from build123d import *

# Parameters (mm, degrees)
F2_DEPTH = 19.05
F3_W     = 247.65
F3_H     = 19.05
F4_DEPTH = 25.4
F6_DEPTH = 25.4


# Not quite as in the source:
# - a variable given as a bare number and used for a length is read in inches; the dataset says mm whatever the document's units were


with BuildPart() as f2:
    # F1 (on Right) → F2 (new body)
    with BuildSketch(Plane.YZ):
        Polygon((-47.625, 142.875), (-47.625, 0), (-47.625, -142.875), (-295.275, -142.875), (-295.275, -244.475), (-47.625, -244.475), (-47.625, -336.55), (47.625, -336.55), (47.625, 0), (47.625, 336.55), (-47.625, 336.55), (-47.625, 244.475), (-295.275, 244.475), (-295.275, 142.875), align=None)
    extrude(amount=F2_DEPTH)

    # F3 (on face) → F4 (cut)
    with BuildSketch(Plane.YZ.offset(19.05)):
        with Locations((-171.45, 193.675)):
            Rectangle(F3_W, F3_H)
    extrude(amount=-F4_DEPTH, mode=Mode.SUBTRACT)

    # F5 (on face) → F6 (cut)
    with BuildSketch(Plane.YZ.offset(19.05)):
        with BuildLine():
            Line((-47.625, 184.15), (-47.625, 203.2))
            ThreePointArc((-47.625, 203.2), (-57.15, 212.725), (-66.675, 203.2))
            Line((-66.675, 203.2), (-66.675, 184.15))
            ThreePointArc((-66.675, 184.15), (-57.15, 174.625), (-47.625, 184.15))
        make_face()
    extrude(amount=-F6_DEPTH, mode=Mode.SUBTRACT)


solid = f2.part
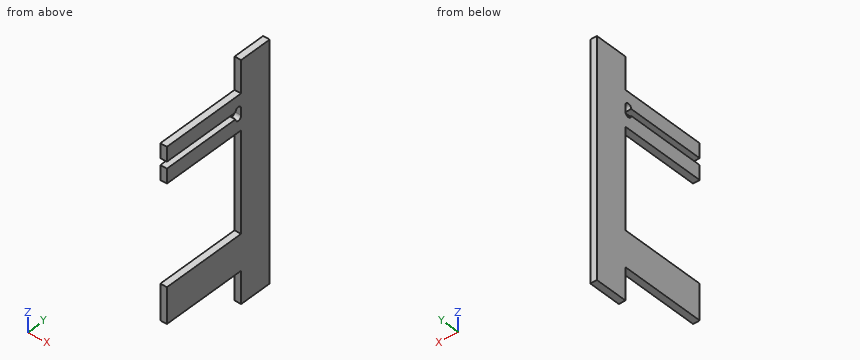
Source: CAD feature listing. Evaluate the final solid. Frame: model axes, mm. Coordinates: 2 decimals unless noted, no trailing zeros. Loops run counter-clockwise (first coordinate to the right, second up) from the corner with the lowest first, then second, coordinate; pieces in that order, holes last. Notation, with made-up numbers: (61.5, 39) - (74.5, 39) arc R13 ccw to (74.5, 61) - close; hole circle Ø6 at (20.25, 29). An arc over 180 degrees is marked (long way). One line per item, written item: value. Start each with the question number.
1. Section A-A (y = -57.15). Return the cut outline in (x, z) (3 decimals), and give its area (3 significant figures).
2. Ray query, L1, parallel to Z at x = 14.25, y = -203.5 (3 decimals); L2, parallel to Y at x = 4, z = 44 (3 decimals); L3, parallel to Y at x = 8.5, z = 211 (3 decimals). Return the intervals inside material, ascending.
3. Section B-B (x = 6.25). Return the cut outline in (y, z) (3 decimals).
4. Contact query for flat-ended pins moving along their axis: P1, Ø1.5, axis at x = 5, y = -119, coming from the +Z side (3 decimals); P2, Ø9.5, axis at x = 9.5, z = 301, coming from the -Y side (3 decimals); P3, Ø5.5, axis at x = 10.5, y = -224.5, coming from the -Z side (3 decimals). Output: stop coordinate, or through.
5. Section C-C (z = 120.5). Return the cut outline in (x, y) (3 decimals), and give its area (3 significant figures).
Verdict:
1. outline: (0, -244.475) - (19.05, -244.475) - (19.05, -142.875) - (0, -142.875) - close; (0, 142.875) - (19.05, 142.875) - (19.05, 174.625) - (0, 174.625) - close; (0, 212.725) - (19.05, 212.725) - (19.05, 244.475) - (0, 244.475) - close
1. area: 3,150 mm2
2. L1: z = -244.475 to -142.875, 142.875 to 184.15, 203.2 to 244.475
2. L2: y = -47.625 to 47.625
2. L3: y = -295.275 to -62.617, -51.683 to 47.625
3. outline: (-295.275, -244.475) - (-47.625, -244.475) - (-47.625, -336.55) - (47.625, -336.55) - (47.625, 336.55) - (-47.625, 336.55) - (-47.625, 244.475) - (-295.275, 244.475) - (-295.275, 203.2) - (-66.675, 203.2) arc R9.525 cw to (-47.625, 203.2) - (-47.625, 184.15) arc R9.525 cw to (-66.675, 184.15) - (-295.275, 184.15) - (-295.275, 142.875) - (-47.625, 142.875) - (-47.625, -142.875) - (-295.275, -142.875) - close
4. P1: stops at z = 244.475
4. P2: stops at y = -47.625
4. P3: stops at z = -244.475
5. outline: (0, -47.625) - (19.05, -47.625) - (19.05, 47.625) - (0, 47.625) - close
5. area: 1,810 mm2
